Part print with two shaded views. Sizes in mm from the minimum x, y, z corner. A direction names the side the tool comes from. Round coordinates to 2 decimals unless told otherwise and drop trailing zeros. Loops run counter-clockwise (first coordinate to the right, second up) from the corner with the lowest first, then second, coordinate; pieces in that order, holes last. Notation, with made-up numbers: (-29, 40) -> (30, 40) arc R11 ccw to (30, 55) -> close; hole circle Ø4 at (79, -29). An arc over 180 degrees is marked (long way). Use a Markdown table: item, result. Add a question column.
Item 1: Cut at A-A, the plane z = 25. List the corners of the cut face in (x, y), plus the area to 4 significant figures.
Item 2: Flat gauge pin, fed straight in: pin 1 (10 mm diameter, centred on x = 9, z = 14, fed in from -Y). Where does the tip first touch, or does it go through?
Item 3: Cut at D-D, the plane z = 37.5. List the corners of the cut face in (x, y), plus the area to 3 significant figures.
Item 4: Cut at B-B, the plane x = 15. List the corners of the cut face in (y, z), plus the area to 3 significant figures.
Item 5: Which spindle directions (+Z, -Z, +X, -X, +Y, -Y) get a long thin tool onto all of the face, cutting with end or side? Do the marked faces 1 and 2. Say none if no direction does.
Item 6: Cut at C-C, the plane y = 1.15. List the corners of the cut face in (x, z), plus the area to 3 significant figures.
Item 7: Probe line 1 (Z direction, x = 15, y = 1.3); line 2 (Z direction, x = 11.25, y = 1.8); line 3 (X direction, y = 1.9, z = 46). List the from-to ranges inside material, lowest first. Write a range as [from, to].
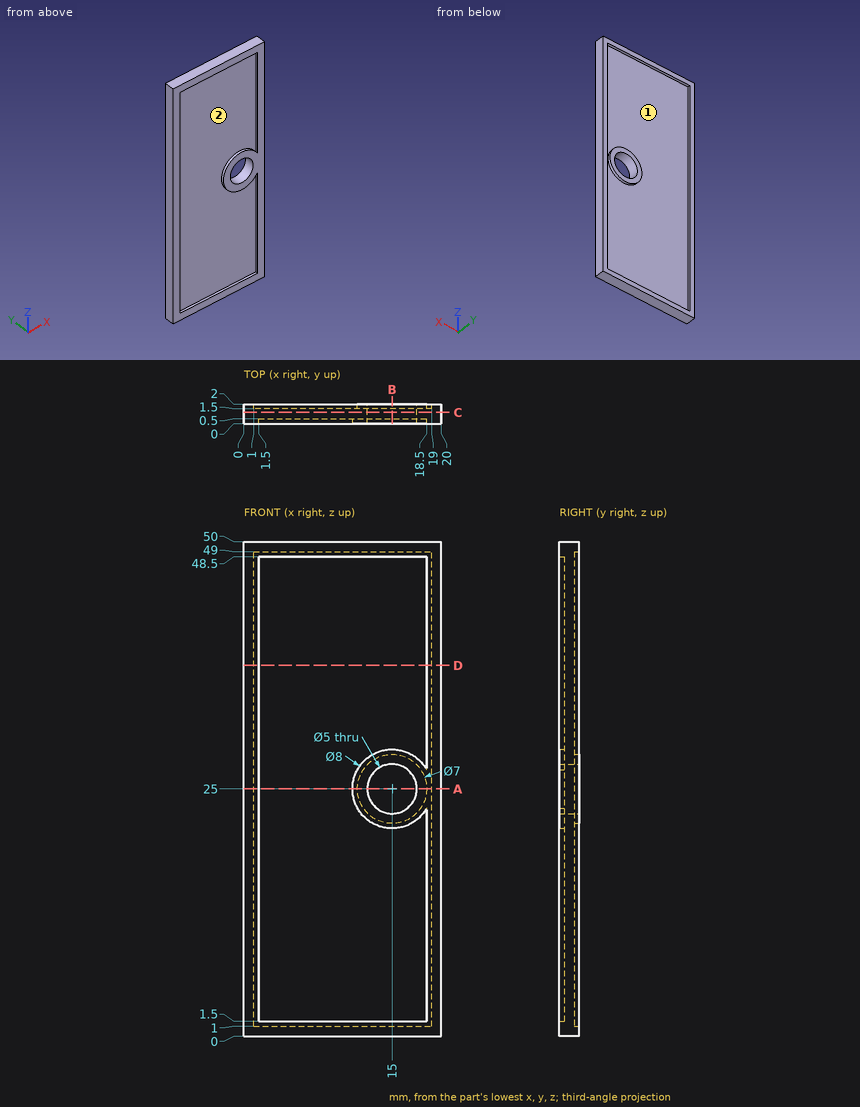
A:
| question | item | result |
|---|---|---|
| 1 | outline | (0, 0) -> (1.5, 0) -> (1.5, 0.5) -> (11, 0.5) -> (11, 0) -> (12.5, 0) -> (12.5, 2) -> (11.5, 2) -> (11.5, 1.5) -> (1, 1.5) -> (1, 2) -> (0, 2) -> close; (17.5, 0) -> (20, 0) -> (20, 2) -> (19, 2) -> (19, 1.5) -> (18.5, 1.5) -> (18.5, 2) -> (17.5, 2) -> close |
| 1 | area | 19.75 mm^2 |
| 2 | pin 1 | stops at y = 0.5 |
| 3 | outline | (0, 0) -> (1.5, 0) -> (1.5, 0.5) -> (18.5, 0.5) -> (18.5, 0) -> (20, 0) -> (20, 2) -> (19, 2) -> (19, 1.5) -> (1, 1.5) -> (1, 2) -> (0, 2) -> close |
| 3 | area | 22.5 mm^2 |
| 4 | outline | (0, 0) -> (2, 0) -> (2, 1) -> (1.5, 1) -> (1.5, 21.5) -> (2, 21.5) -> (2, 22.5) -> (0, 22.5) -> (0, 21) -> (0.5, 21) -> (0.5, 1.5) -> (0, 1.5) -> close; (0, 27.5) -> (2, 27.5) -> (2, 28.5) -> (1.5, 28.5) -> (1.5, 49) -> (2, 49) -> (2, 50) -> (0, 50) -> (0, 48.5) -> (0.5, 48.5) -> (0.5, 29) -> (0, 29) -> close |
| 4 | area | 50.0 mm^2 |
| 5 | face 1 | +Y |
| 5 | face 2 | -Y |
| 6 | outline | (0, 0) -> (20, 0) -> (20, 50) -> (0, 50) -> close; hole circle Ø5 at (15, 25) |
| 6 | area | 980 mm^2 |
| 7 | line 1 | z = [0, 22.5], [27.5, 50] |
| 7 | line 2 | z = [0, 1], [49, 50] |
| 7 | line 3 | x = [0, 1], [19, 20] |
